Geometry check sheet. Reference: the model listing, model coordinates, mm. A direction names the side the tool comes from. Round coordinates to 2 decimals unless told otherwise and drop trailing zeros. Order: outer loops, then holes, each group sorted by start corner. A loop starts at its lowest first (then second) coordinate and runs counter-clockwise, first axis right, second up. Notation, with made-up numbers: (73, 1) -> (83, 1) arc R32 ccw to (83, 36) -> close; hole circle Ø2 at (-39, 40.5). An arc over 180 degrees is marked (long way). Answer as a JSON object with one key per item and string values. Group by question number.
from build123d import *

# Parameters (mm, degrees)
SKETCH1_R          = 14.25
EXTRUDE1_DEPTH     = 2.2
SKETCH2_R          = 11
EXTRUDE2_DEPTH     = 0.5
SKETCH3_R          = 10
EXTRUDE3_DEPTH     = 4
SKETCH4_R          = 8.5
CUT_EXTRUDE1_DEPTH = 22.23711374


with BuildPart() as part:
    # Sketch1 → Extrude1 (new body)
    with BuildSketch(Plane.XY):
        Circle(SKETCH1_R)
    extrude(amount=EXTRUDE1_DEPTH)

    # Sketch2 → Extrude2 (add)
    with BuildSketch(Plane.XY.offset(2.2)):
        Circle(SKETCH2_R)
    extrude(amount=EXTRUDE2_DEPTH)

    # Sketch3 → Extrude3 (add)
    with BuildSketch(Plane.XY.offset(2.7)):
        Circle(SKETCH3_R)
    extrude(amount=EXTRUDE3_DEPTH)

    # Sketch4 → Cut-Extrude1 (cut, through all)
    with BuildSketch(Plane.XY.offset(6.7)):
        Circle(SKETCH4_R)
    extrude(amount=-CUT_EXTRUDE1_DEPTH, mode=Mode.SUBTRACT)


solid = part.part
Item 1: Sectioned sample at A-A, the plane y = 0. Enter the section's corners in (x, z), then the cut area to 3 significant figures.
Item 2: Sectioned sample at D-D, the plane x = 12. Enter the section's corners in (y, z).
Item 3: Depth check by flat-ended pin: pin 1 Ø1 at (x, z) = (3.5, 5.5) entering from +Y; pin 2 Ø1.5 at (y, z) = (1, 6) entering from -X; pin 3 Ø1 at (x, z) = (4, 2.5) entering from -Y; pin 4 Ø13.5 at (x, y) = (0, 0) entering from +Z. Enter the tip coordinate at first touch or a pass-through.
Item 4: Set-up check for faces 4 (the cylindrical face through (13.163, -5.458, 1.085)), 5 (the cylindrical face through (-2.17, -9.76, 4.67)): record each of +Z, -Z, +X, -X, +Y, -Y from which the full face is reachable in a straight line by a thin tool's end or side.
Item 5: Mould release check, pull along X, two halves, no side actions. Record for faces 1 (the cylindrical face through (-2.38, -10.74, 2.45)), 2 (the flat face through (6.13, -6.13, 0)), 3 (the cylindrical face through (4.57, 7.167, 3.397)): pulls with the +X half, pulls with the -X half, needs draft (parallel to the pull), parting line crosses it, or undercut.
Item 6: Thickness scan on L1, parallel to Y at x = 0, z = 3; L2, parallel to X at y = -2.25, z = 4.5; L3, parallel to X at y = -4.25, z = 6. Record the ranges inside material, lowest first.
Item 7: Sectioned sample at C-C, the plane z = 5.5. Enter the section's corners in (x, y).
Result:
{
 "1": {"outline": "(-14.25, 0) -> (-8.5, 0) -> (-8.5, 6.7) -> (-10, 6.7) -> (-10, 2.7) -> (-11, 2.7) -> (-11, 2.2) -> (-14.25, 2.2) -> close; (8.5, 0) -> (14.25, 0) -> (14.25, 2.2) -> (11, 2.2) -> (11, 2.7) -> (10, 2.7) -> (10, 6.7) -> (8.5, 6.7) -> close", "area": "39.8 mm2"},
 "2": {"outline": "(-7.69, 0) -> (7.69, 0) -> (7.69, 2.2) -> (-7.69, 2.2) -> close"},
 "3": {"pin 1": "stops at y = 9.54", "pin 2": "stops at x = -10", "pin 3": "stops at y = -13.79", "pin 4": "passes through"},
 "4": {"face 4": "+Z, -Z", "face 5": "+Z"},
 "5": {"face 1": "parting line crosses it", "face 2": "needs draft", "face 3": "undercut"},
 "6": {"L1": "y = -10 to -8.5, 8.5 to 10", "L2": "x = -9.74 to -8.2, 8.2 to 9.74", "L3": "x = -9.05 to -7.36, 7.36 to 9.05"},
 "7": {"outline": "circle Ø20 at (0, 0); hole circle Ø17 at (0, 0)"}
}
